from build123d import *

# Parameters (mm, degrees)
SKETCH1_W                   = 6.35
SKETCH1_H                   = 165
BOSS_EXTRUDE1_DEPTH         = 370
F_1_4_0_25_DIAMETER_HOLE1_D = 6.35
CUT_EXTRUDE1_DEPTH          = 380.139252122


with BuildPart() as part:
    # Sketch1 → Boss-Extrude1 (new body)
    with BuildSketch(Plane(origin=(0, 0, 0), x_dir=(1, 0, 0), z_dir=(0, 1, 0))):
        with Locations((3.175, 0)):
            Rectangle(SKETCH1_W, SKETCH1_H)
    extrude(amount=BOSS_EXTRUDE1_DEPTH)

    # 1/4 (0.25) Diameter Hole1 (through all)
    with Locations(Plane(origin=(6.35, 0, 0), x_dir=(0, 0, -1), z_dir=(1, 0, 0))):
        with Locations((0, 354.147260033)):
            Hole(F_1_4_0_25_DIAMETER_HOLE1_D / 2)

    # Sketch4 → Cut-Extrude1 (cut, through all)
    with BuildSketch(Plane(origin=(6.35, 0, 0), x_dir=(0, 0, -1), z_dir=(1, 0, 0))):
        Polygon((-22.5, 370), (-82.5, 220), (-82.5, 370), align=None)
        Polygon((82.5, 370), (22.5, 370), (82.5, 220), align=None)
    extrude(amount=-CUT_EXTRUDE1_DEPTH, mode=Mode.SUBTRACT)


solid = part.part
Check sheet for the modelled part. Datum: model origin and axes. Units: mm. Round coordinates to 2 decimals unless told otherwise and drop trailing zeros. Write each loop counter-clockwise with the first axis right and the second up, starting at its lowest first coordinate (ties: lowest second). Pieces come first, ordered by that corner, then holes. Notation, with made-up numbers: (6, 86.5) -> (59, 86.5) arc R20 ccw to (59, 107.5) -> close; hole circle Ø9 at (-17, 72). An arc over 180 degrees is marked (long way). Answer as CSV lines item,"result". Start each with the question number.
1) Release check for a two-part mould opening along Z. For faces 1 (the cylindrical face through (3.131, 357.295, -0.413)), 2 (the flat face through (3.2, 296, -52.1)), 3 (the flat face through (0, 141, 1)) record: pulls with the +Z half, pulls with the -Z half, needs draft (parallel to the pull), parting line crosses it, or undercut.
2) Section check B-B on z = 38. Enter the section's corners in (x, y).
3) Section check A-A on x = 4.5. Enter the section's corners in (y, z) (3 decimals).
4) Material ranges on line 1 (Y direction, x = 3.25, z = 0); line 2 (Z direction, x = 5.5, y = 264); line 3 (Z direction, x = 6.25, y = 233), recorded low to high. Write a range as from..to.
5) Section check C-C on y = 253. Enter the section's corners in (x, z), and give its area (3 significant figures).
Found:
1,face 1,"undercut"
1,face 2,"pulls with the -Z half"
1,face 3,"needs draft"
2,outline,"(0, 0) -> (6.35, 0) -> (6.35, 331.25) -> (0, 331.25) -> close"
3,outline,"(0, -82.5) -> (220, -82.5) -> (370, -22.5) -> (370, 22.5) -> (220, 82.5) -> (0, 82.5) -> close; hole circle Ø6.35 at (354.147, 0)"
4,line 1,"y = 0..350.97, 357.32..370"
4,line 2,"z = -64.9..64.9"
4,line 3,"z = -77.3..77.3"
5,outline,"(0, -69.3) -> (6.35, -69.3) -> (6.35, 69.3) -> (0, 69.3) -> close"
5,area,"880 mm^2"
